Could you check a few things on this model? Use its own coordinates, in mm. Face numbers are marked on the shaded views. A direction names the side the tool comes from. Give positions to 0.01 mm unless a question says otherwise; leave off trailing zeros. Write each loop counter-clockwise with the first axis right and the second up, starting at its lowest first coordinate (ties: lowest second). Pieces come first, ordered by that corner, then holes. Notation, with made-up numbers: (71, 20) - (104, 20) arc R27 cw to (104, 50) - close; hole circle Ø1 at (-9, 27.25). An arc over 180 degrees is marked (long way). Write item = value, one per line.
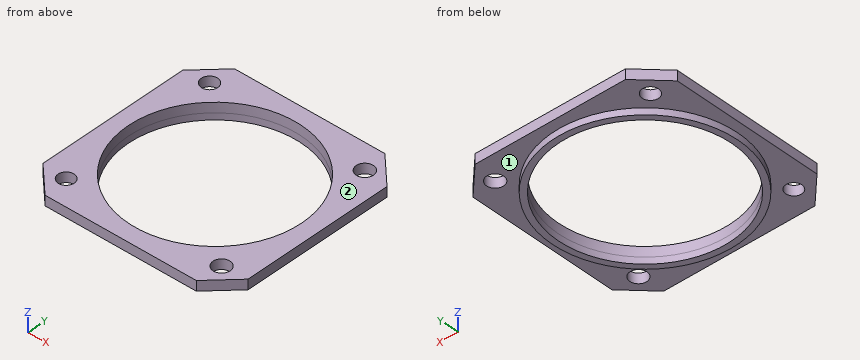
Autodesk Inventor part; units mm, degrees
ref_plane "YZ Plane" through (0, 0, 0) normal (1, 0, 0) x (0, 1, 0)
ref_plane "XZ Plane" through (0, 0, 0) normal (0, 1, 0) x (-1, 0, 0)
ref_plane "XY Plane" through (0, 0, 0) normal (0, 0, 1) x (1, 0, 0)
ref_plane "Arbeitsebene1" through (-58.716, -54.45, 1.8) normal (0, 0, 1) x (1, 0, 0)
sketch "Skizze1" plane through (-58.716, -54.45, 0) normal (0, 0, 1) x (1, 0, 0)
  circle A0 centre (-11.3643, -15.5584) radius 13.0833
  line L0 (4.216, -27.049) -> (4.216, -4.234)
  line L1 (4.216, -4.234) -> (0, 0)
  line L2 (0, 0) -> (-22.71, 0)
  line L3 (-22.71, 0) -> (-26.784, -4.092)
  line L4 (-26.784, -4.092) -> (-26.784, -27.049)
  line L5 (-26.784, -27.049) -> (-22.71, -31.14)
  line L6 (-22.71, -31.14) -> (0.142, -31.14)
  line L7 (0.142, -31.14) -> (4.216, -27.049)
  circle A1 centre (0.4286, -27.2971) radius 1.2941
  circle A2 centre (0.4173, -3.7431) radius 1.3039
  circle A3 centre (-23.0288, -3.7639) radius 1.2464
  circle A4 centre (-23.0166, -27.3387) radius 1.2172
  point P0 (58.716, 54.45)
extrude "Extrusion1" add sketch "Skizze1" along normal blind 1.5
sketch "Skizze2" plane through (-58.716, -54.45, 0) normal (0, 0, -1) x (-1, 0, 0)
  circle A0 centre (11.3643, -15.5584) radius 13.0833
  circle A1 centre (11.3643, -15.5584) radius 14
  point P0 (-58.716, 54.45)
  dimension "d2" = 28
extrude "Extrusion2" add sketch "Skizze2" along normal blind 1
properties part number "Pump_Lid"
1. I need wall thicknesses on line 1 (Y direction, x = -70, z = 1.35); line 2 (X direction, y = -73, z = 0.6); line 3 (X direction, y = -75, z = -0.2). Which ranges of each line are inside material? Lowest first, please.
Filled sheet:
line_1 = -85.59 to -83.09, -56.93 to -54.45
line_2 = -85.5 to -82.82, -57.34 to -54.5
line_3 = -83.16 to -82.17, -57.99 to -57
2. If we section it at D-D, the plane z = 0.45: Please give me the cut outline in (x, y), and give its area (3 significant figures).
Filled sheet:
outline = (-85.5, -81.5) - (-81.43, -85.59) - (-58.57, -85.59) - (-54.5, -81.5) - (-54.5, -58.68) - (-58.72, -54.45) - (-81.43, -54.45) - (-85.5, -58.54) - close; hole circle Ø26.17 at (-70.08, -70.01); hole circle Ø2.49 at (-81.74, -58.21); hole circle Ø2.43 at (-81.73, -81.79); hole circle Ø2.61 at (-58.3, -58.19); hole circle Ø2.59 at (-58.29, -81.75)
area = 374 mm2
3. Which directions (+Z, -Z, +X, -X, +Y, -Y) give clear straight access to the entire face, cutting with the end or side of a thin tool? Please do the marked faces 1 and 2.
Filled sheet:
face_1 = -Z
face_2 = +Z, +X, -X, +Y, -Y
4. If we section it at B-B, the plane y = -64: Please give me the cut outline in (x, z).
Filled sheet:
outline = (-85.5, 0) - (-82.73, 0) - (-82.73, -1) - (-81.7, -1) - (-81.7, 1.5) - (-85.5, 1.5) - close; (-58.46, -1) - (-57.44, -1) - (-57.44, 0) - (-54.5, 0) - (-54.5, 1.5) - (-58.46, 1.5) - close
5. For pin 1 (2 mm diameter, centred on x = -81.73, y = -81.79, fed in from -Z); pin 2 (4 mm diameter, centred on x = -81.74, y = -58.21, fed in from -Z), each with a flat end and sliding along its axis, tell me the tip position at first contact or that it passes through.
Filled sheet:
pin_1 = through
pin_2 = 0
6. If we section it at A-A, the plane x = -81: Please give me the cut outline in (y, z), and give its area (3 significant figures).
Filled sheet:
outline = (-85.59, 0) - (-82.76, 0) - (-82.76, 1.5) - (-85.59, 1.5) - close; (-80.82, 0) - (-78.77, 0) - (-78.77, -1) - (-77.21, -1) - (-77.21, 1.5) - (-80.82, 1.5) - close; (-62.8, -1) - (-61.25, -1) - (-61.25, 0) - (-59.21, 0) - (-59.21, 1.5) - (-62.8, 1.5) - close; (-57.21, 0) - (-54.45, 0) - (-54.45, 1.5) - (-57.21, 1.5) - close
area = 22.3 mm2
7. If we section it at C-C, the plane x = -74.5: Please give me the cut outline in (y, z).
Filled sheet:
outline = (-85.59, 0) - (-83.29, 0) - (-83.29, -1) - (-82.32, -1) - (-82.32, 1.5) - (-85.59, 1.5) - close; (-57.69, -1) - (-56.72, -1) - (-56.72, 0) - (-54.45, 0) - (-54.45, 1.5) - (-57.69, 1.5) - close
